```python
from build123d import *

# Parameters (mm, degrees)
SKETCH_1_R      = 3
EXTRUDE_1_DEPTH = 8
SKETCH_2_R      = 3
SKETCH_2_R_2    = 1.8
EXTRUDE_2_DEPTH = 4


with BuildPart() as part:
    # 草图1 → 凸台-拉伸1 (new body)
    with BuildSketch(Plane(origin=(0, 0, 0), x_dir=(1, 0, 0), z_dir=(0, 1, 0))):
        Circle(SKETCH_1_R)
        with BuildLine():
            ThreePointArc((1.24498996, -1.3), (0, 1.8), (-1.24498996, -1.3))
            Line((-1.24498996, -1.3), (1.24498996, -1.3))
        make_face(mode=Mode.SUBTRACT)
    extrude(amount=EXTRUDE_1_DEPTH)

    # 草图2 → 凸台-拉伸2 (add)
    with BuildSketch(Plane(origin=(0, 8, 0), x_dir=(1, 0, 0), z_dir=(0, 1, 0))):
        Circle(SKETCH_2_R)
        Circle(SKETCH_2_R_2, mode=Mode.SUBTRACT)
    extrude(amount=EXTRUDE_2_DEPTH)


solid = part.part
```
Input: part model. Units: mm. Frame: model coordinates. Round coordinates to 2 decimals unless told otherwise and drop trailing zeros. Loops run counter-clockwise (first coordinate to the right, second up) from the corner with the lowest first, then second, coordinate; pieces in that order, holes last. Notation, with made-up numbers: (44, 59) -> (97, 59) arc R30 cw to (97, 85) -> close; hole circle Ø5 at (26.5, -35.5). An arc over 180 degrees is marked (long way). Use one line per item in the form item = value. Start each with the question number.
Item 1: Mould query, pull axis X, two halves, no side actions, for faces 1 (the face through (0, 4, 1.3)), 2 (the face through (-3, 6, 0)), 3 (the face through (0, 12, 2)). Classes: pulls with the +X half, pulls with the -X half, needs draft (parallel to the pull), parting line crosses it, or undercut.
Item 2: Section query A-A on z = 0. Return the cut outline in (x, y).
Item 3: Section query D-D on x = 1.1. Return the cut outline in (y, z).
Item 4: Contact query for flat-ended pins moving along their axis: pin 1 Ø0.6 at (x, z) = (-0.5, 1.5) entering from +Y; pin 2 Ø1 at (y, z) = (10, -2.5) entering from +X; pin 3 Ø1 at (y, z) = (10, -1) entering from -X. Output: stop coordinate, or through.
Item 5: Section query C-C on y = 8.75. Return the cut outline in (x, z).
Item 6: Section query B-B on x = 0. Return the cut outline in (y, z).
Item 7: Material intervals for L1, parallel to Z at x = 0.1, y = 11; L2, parallel to Z at x = 0, y = 2.5, sorted ascending. Write a range as from..to.
Ans:
q1.face_1 = undercut
q1.face_2 = parting line crosses it
q1.face_3 = needs draft
q2.outline = (-3, 0) -> (-1.8, 0) -> (-1.8, 12) -> (-3, 12) -> close; (1.8, 0) -> (3, 0) -> (3, 12) -> (1.8, 12) -> close
q3.outline = (0, -2.79) -> (12, -2.79) -> (12, -1.42) -> (0, -1.42) -> close; (0, 1.3) -> (8, 1.3) -> (8, 1.42) -> (12, 1.42) -> (12, 2.79) -> (0, 2.79) -> close
q4.pin_1 = 12
q4.pin_2 = 2.24
q4.pin_3 = -2.96
q5.outline = circle Ø6 at (0, 0); hole circle Ø3.6 at (0, 0)
q6.outline = (0, -3) -> (12, -3) -> (12, -1.8) -> (0, -1.8) -> close; (0, 1.3) -> (8, 1.3) -> (8, 1.8) -> (12, 1.8) -> (12, 3) -> (0, 3) -> close
q7.L1 = -3..-1.8, 1.8..3
q7.L2 = -3..-1.8, 1.3..3
